The model under review builds one solid part; all positions refer to its coordinate system, in mm. A direction names the side the tool comes from. Round coordinates to 2 decimals unless told otherwise and drop trailing zeros. Loops run counter-clockwise (first coordinate to the right, second up) from the corner with the lowest first, then second, coordinate; pieces in that order, holes last. Notation, with made-up numbers: M -7.75,54.25 L 15.25,54.25 A16 ccw 15.25,78.25 Z; hole C 72,86 d9. An arc over 180 degrees is marked long. Return JSON: item names as keys, results as strings. Group by question number.
Q1. Draft analysis for pull direction Z (two halves, no side actions). For faces 1 (the face through (-23, 24, -24)), 2 (the face through (-50.8, 175, -13)), 3 (the face through (-25, 175, -1.905)), state which applies: pulls with the +Z half, pulls with the -Z half, needs draft (parallel to the pull), parting line crosses it, or undercut.
Q2. Consider section A-A (z = -14.25). State the section outline as (x, y) points (3 decimals).
Q3. Consider section C-C (y = 244.5). State the section outline as (x, z) points (3 decimals).
Q4. Clearance check with a flat-ended pin moving along its axis: pin 1 Ø23.5 at (x, y) = (-16, 102.5) entering from +Z. State where the tip first meets the part, or that it passes through.
Q5. Consider section B-B (x = -29). State the section outline as (y, z) points (3 decimals).
Q6. To check wall thickness, follow line 1 along X through (y, z) = (209, -9.5) (3 decimals); line 2 along Z through (x, y) = (-37, 223) (3 decimals); line 3 along Z through (x, y) = (-6, 336.5) (3 decimals). State the ranges of each line that lie inside material, in increasing order.
Q7. For faces 4 (the face through (-23.4, 331.6, -24)), 5 (the face through (-48.895, 175, -13)), list the 3-axis set-ups (+Z, -Z, +X, -X, +Y, -Y) from which the entire face can be reached by the end or side of a thin tool; tool diameter is ignored.
Autodesk Inventor part; units mm, degrees
ref_plane "YZ Plane" through (0, 0, 0) normal (1, 0, 0) x (0, 1, 0)
ref_plane "XZ Plane" through (0, 0, 0) normal (0, 1, 0) x (-1, 0, 0)
ref_plane "XY Plane" through (0, 0, 0) normal (0, 0, 1) x (1, 0, 0)
sketch "Sketch1" plane through (0, 0, 0) normal (0, 1, 0) x (-1, 0, 0)
  line L0 (0, 0) -> (50.8, 0)
  line L1 (50.8, 0) -> (50.8, -25.4)
  line L2 (50.8, -25.4) -> (0, -25.4)
  line L3 (0, -25.4) -> (0, 0)
  dimension "d0" = 50.8
  dimension "d1" = 25.4
extrude "Extrusion1" add sketch "Sketch1" along normal blind 355.6
sketch "Sketch3" plane through (0, 0, 0) normal (1, 0, 0) x (0, 0, -1)
  line L0 (25.4, 0) -> (0, 0)
  line L1 (25.4, 0) -> (25.4, 25.4)
  line L2 (25.4, 0) -> (25.4, 355.6)
  line L3 (0, 0) -> (0, 355.6)
  line L4 (25.4, 25.4) -> (0, 0)
  line L5 (0, 177.8) -> (104.5089, 177.8)
  line L6 (0, 0) -> (25.4, 0)
  line L7 (25.4, 355.6) -> (0, 355.6)
  line L8 (25.4, 355.6) -> (25.4, 330.2)
  line L9 (25.4, 330.2) -> (0, 355.6)
  line L10 (0, 355.6) -> (25.4, 355.6)
  dimension "d4" = 25.4
shell "Shell1" thickness 1.905 removed faces 2 at (-16.9333, 0, -16.9333) at (-16.9333, 355.6, -16.9333)
extrude "Extrusion2" cut sketch "Sketch3" against normal blind 355.6 contours L0 L4 L1 | L7 L2 L9
properties part number "graber back peice"
Values:
{
 "1": {"face 1": "pulls with the -Z half", "face 2": "needs draft", "face 3": "undercut"},
 "2": {"outline": "M -50.8,14.25 L -48.895,14.25 L -48.895,341.35 L -50.8,341.35 Z; M -1.905,14.25 L 0,14.25 L 0,341.35 L -1.905,341.35 Z"},
 "3": {"outline": "M -50.8,-25.4 L 0,-25.4 L 0,0 L -50.8,0 Z; hole M -48.895,-23.495 L -1.905,-23.495 L -1.905,-1.905 L -48.895,-1.905 Z"},
 "4": {"pin 1": "stops at z = 0"},
 "5": {"outline": "M 0,0 L 1.905,-1.905 L 353.695,-1.905 L 355.6,0 Z; M 23.495,-23.495 L 25.4,-25.4 L 330.2,-25.4 L 332.105,-23.495 Z"},
 "6": {"line 1": "x = -50.8 to -48.895, -1.905 to 0", "line 2": "z = -25.4 to -23.495, -1.905 to 0", "line 3": "z = -1.905 to 0"},
 "7": {"face 4": "-Z, +X, -X, +Y", "face 5": "+Y, -Y"}
}
